Work out the finished part from the listing and answer in its coordinate system (mm). A direction names the side the tool comes from. Give positions to 0.01 mm unless a question says otherwise; leave off trailing zeros. Write each loop counter-clockwise with the first axis right and the second up, starting at its lowest first coordinate (ties: lowest second). Pieces come first, ordered by that corner, then holes. Notation, with made-up numbers: (6, 64.25) -> (16, 64.25) arc R20 ccw to (16, 101.25) -> close; hole circle Ø11 at (17, 82). An arc over 180 degrees is marked (long way). Use a Markdown table: item, result. Add a question column.
Q1. Section D-D, the plane y = 0.9 is taken. State how many separate pieces and enclosed holes the cut face has, plus the area to 3 significant figures.
Q2. Section B-B, the plane z = -9.25 is taken. Give the vertices of the cut face in (x, y) (3 decimals).
Q3. Section A-A, the plane z = -6.35 is taken. Give the vertices of the cut face in (x, y) (3 decimals), plus the area to 3 significant figures.
Q4. Consider line 1 (X direction, y = 1, z = -3.5) (3 decimals); line 2 (Z direction, x = 34, y = 0.9); line 3 (X direction, y = 1.85, z = -2) (3 decimals). Determine where each line is inside the solid, lowest interval first.
Q5. For a pull along Z with two mould halves and no side action, classify faces 3 (the face through (11.635, 1, -5)), 4 (the face through (28, 1, 0)), 5 (the face through (0.724, 1.006, -11.936)) as pulls with the +Z half, pulls with the -Z half, needs draft (parallel to the pull), parting line crosses it, or undercut.
Q6. For faces 1 (the face through (31.955, 1, -5)), 2 (the face through (56.286, 1.006, -11.976)), determine the directions among +Z, -Z, +X, -X, +Y, -Y from which every point of the face is accessible in a straight line to the end or side of a thin tool.
Q7. Section C-C, the plane x = 12.5 is taken. Give the vertices of the cut face in (y, z).
from build123d import *

# Parameters (mm, degrees)
SKETCH1_W           = 57.05
SKETCH1_H           = 12.7
SKETCH1_R           = 1.89865
BOSS_EXTRUDE1_DEPTH = 1.984375
CUT_EXTRUDE1_REACH  = 60.48
FILLET1_R           = 2.54


with BuildPart() as part:
    # Sketch1 → Boss-Extrude1 (new body)
    with BuildSketch(Plane(origin=(0, 0, 0), x_dir=(1, 0, 0), z_dir=(0, 1, 0))):
        with Locations((28.525, 6.35)):
            Rectangle(SKETCH1_W, SKETCH1_H)
        with Locations(Location((52.2875, 6.35, 0), (0, 0, 270))):
            Circle(SKETCH1_R, mode=Mode.SUBTRACT)
        with Locations(Location((4.7625, 6.35, 0), (0, 0, 270))):
            Circle(SKETCH1_R, mode=Mode.SUBTRACT)
    extrude(amount=BOSS_EXTRUDE1_DEPTH)

    # Sketch2 → Cut-Extrude1 (cut, up to next)
    with BuildSketch(Plane(origin=(0, 1.984375, 0), x_dir=(1, 0, 0), z_dir=(0, 1, 0)), mode=Mode.PRIVATE) as cut_extrude1_sk1:
        Polygon((17.475, 1.23), (11.635, 1.23), (11.635, 9.808717093), (13.29671726, 11.47), (15.81328274, 11.47), (17.475, 9.808717093), align=None)
    cut_extrude1_tool1 = extrude(cut_extrude1_sk1.sketch, amount=-CUT_EXTRUDE1_REACH, mode=Mode.PRIVATE) & part.part
    # Sketch2 → Cut-Extrude1 (cut, up to next)
    with BuildSketch(Plane(origin=(0, 1.984375, 0), x_dir=(1, 0, 0), z_dir=(0, 1, 0)), mode=Mode.PRIVATE) as cut_extrude1_sk2:
        Polygon((45.415, 1.23), (39.575, 1.23), (39.575, 9.808717093), (41.23671726, 11.47), (43.75328274, 11.47), (45.415, 9.808717093), align=None)
    cut_extrude1_tool2 = extrude(cut_extrude1_sk2.sketch, amount=-CUT_EXTRUDE1_REACH, mode=Mode.PRIVATE) & part.part
    # Sketch2 → Cut-Extrude1 (cut, up to next)
    with BuildSketch(Plane(origin=(0, 1.984375, 0), x_dir=(1, 0, 0), z_dir=(0, 1, 0)), mode=Mode.PRIVATE) as cut_extrude1_sk3:
        Polygon((25.095, 1.23), (19.255, 1.23), (19.255, 9.808717093), (20.91671726, 11.47), (23.43328274, 11.47), (25.095, 9.808717093), align=None)
    cut_extrude1_tool3 = extrude(cut_extrude1_sk3.sketch, amount=-CUT_EXTRUDE1_REACH, mode=Mode.PRIVATE) & part.part
    # Sketch2 → Cut-Extrude1 (cut, up to next)
    with BuildSketch(Plane(origin=(0, 1.984375, 0), x_dir=(1, 0, 0), z_dir=(0, 1, 0)), mode=Mode.PRIVATE) as cut_extrude1_sk4:
        Polygon((37.795, 1.23), (31.955, 1.23), (31.955, 9.808717093), (33.61671726, 11.47), (36.13328274, 11.47), (37.795, 9.808717093), align=None)
    cut_extrude1_tool4 = extrude(cut_extrude1_sk4.sketch, amount=-CUT_EXTRUDE1_REACH, mode=Mode.PRIVATE) & part.part
    add(cut_extrude1_tool1.solids().sort_by_distance((14.555, 1.984375, -6.12901))[0], mode=Mode.SUBTRACT)
    add(cut_extrude1_tool2.solids().sort_by_distance((42.495, 1.984375, -6.12901))[0], mode=Mode.SUBTRACT)
    add(cut_extrude1_tool3.solids().sort_by_distance((22.175, 1.984375, -6.12901))[0], mode=Mode.SUBTRACT)
    add(cut_extrude1_tool4.solids().sort_by_distance((34.875, 1.984375, -6.12901))[0], mode=Mode.SUBTRACT)

    # Fillet1
    fillet1_edges = [part.edges().sort_by_distance(p)[0] for p in [
        (0, 0.9921875, -12.7),
        (57.05, 0.9921875, -12.7),
        (57.05, 0.9921875, 0),
        (0, 0.9921875, 0),
    ]]
    fillet(fillet1_edges, radius=FILLET1_R)


solid = part.part
Result set:
| question | item | result |
|---|---|---|
| 1 | separate pieces | 1 |
| 1 | enclosed holes | 6 |
| 1 | area | 468 mm2 |
| 2 | outline | (0, 0) -> (11.635, 0) -> (11.635, 1.984) -> (0, 1.984) -> close; (17.475, 0) -> (19.255, 0) -> (19.255, 1.984) -> (17.475, 1.984) -> close; (25.095, 0) -> (31.955, 0) -> (31.955, 1.984) -> (25.095, 1.984) -> close; (37.795, 0) -> (39.575, 0) -> (39.575, 1.984) -> (37.795, 1.984) -> close; (45.415, 0) -> (57.05, 0) -> (57.05, 1.984) -> (45.415, 1.984) -> close |
| 3 | outline | (0, 0) -> (2.864, 0) -> (2.864, 1.984) -> (0, 1.984) -> close; (6.661, 0) -> (11.635, 0) -> (11.635, 1.984) -> (6.661, 1.984) -> close; (17.475, 0) -> (19.255, 0) -> (19.255, 1.984) -> (17.475, 1.984) -> close; (25.095, 0) -> (31.955, 0) -> (31.955, 1.984) -> (25.095, 1.984) -> close; (37.795, 0) -> (39.575, 0) -> (39.575, 1.984) -> (37.795, 1.984) -> close; (45.415, 0) -> (50.389, 0) -> (50.389, 1.984) -> (45.415, 1.984) -> close; (54.186, 0) -> (57.05, 0) -> (57.05, 1.984) -> (54.186, 1.984) -> close |
| 3 | area | 51.8 mm2 |
| 4 | line 1 | x = 0 to 11.635, 17.475 to 19.255, 25.095 to 31.955, 37.795 to 39.575, 45.415 to 57.05 |
| 4 | line 2 | z = -12.7 to -11.47, -1.23 to 0 |
| 4 | line 3 | x = 0.058 to 11.635, 17.475 to 19.255, 25.095 to 31.955, 37.795 to 39.575, 45.415 to 56.992 |
| 5 | face 3 | undercut |
| 5 | face 4 | pulls with the +Z half |
| 5 | face 5 | pulls with the -Z half |
| 6 | face 1 | +Y, -Y |
| 6 | face 2 | -Z, +X, +Y, -Y |
| 7 | outline | (0, -12.7) -> (1.98, -12.7) -> (1.98, -10.67) -> (0, -10.67) -> close; (0, -1.23) -> (1.98, -1.23) -> (1.98, 0) -> (0, 0) -> close |
